from build123d import *

# Parameters (mm, degrees)
F1_DEPTH = 1


with BuildPart() as f1:
    # F0 (on Front) → F1 (new body)
    with BuildSketch(Plane.XZ):
        with BuildLine():
            Line((18.708066, 12.50033), (22.98097, 22.98097))
            Line((22.98097, 22.98097), (12.437212, 18.613602))
            Line((12.437212, 18.613602), (12.437212, 30.026085))
            Line((12.437212, 30.026085), (4.315137, 22.082337))
            Line((4.315137, 22.082337), (0, 32.5))
            Line((0, 32.5), (-4.371889, 22.071171))
            Line((-4.371889, 22.071171), (-12.359057, 30.058339))
            ThreePointArc((-12.359057, 30.058339), (-12.437212, 30.026085), (-12.515282, 29.993628))
            Line((-12.515282, 29.993628), (-12.515282, 18.730443))
            Line((-12.515282, 18.730443), (-22.921108, 23.040677))
            ThreePointArc((-22.921108, 23.040677), (-22.979929, 22.982012), (-23.0386, 22.923195))
            Line((-23.0386, 22.923195), (-18.623445, 12.626056))
            Line((-18.623445, 12.626056), (-29.947166, 12.626056))
            ThreePointArc((-29.947166, 12.626056), (-30.026085, 12.437212), (-30.103813, 12.247874))
            Line((-30.103813, 12.247874), (-22.096734, 4.240795))
            Line((-22.096734, 4.240795), (-32.499928, -0.068349))
            Line((-32.499928, -0.068349), (-22.067669, -4.389532))
            Line((-22.067669, -4.389532), (-30.052174, -12.374038))
            ThreePointArc((-30.052174, -12.374038), (-30.026085, -12.437212), (-29.999862, -12.50033))
            Line((-29.999862, -12.50033), (-18.708066, -12.50033))
            Line((-18.708066, -12.50033), (-23.02925, -22.93259))
            ThreePointArc((-23.02925, -22.93259), (-22.98097, -22.98097), (-22.93259, -23.02925))
            Line((-22.93259, -23.02925), (-12.50033, -18.708066))
            Line((-12.50033, -18.708066), (-12.50033, -29.999862))
            ThreePointArc((-12.50033, -29.999862), (-12.437212, -30.026085), (-12.374038, -30.052174))
            Line((-12.374038, -30.052174), (-4.389532, -22.067669))
            Line((-4.389532, -22.067669), (-0.068349, -32.499928))
            ThreePointArc((-0.068349, -32.499928), (0, -32.5), (0.068349, -32.499928))
            Line((0.068349, -32.499928), (4.389532, -22.067669))
            Line((4.389532, -22.067669), (12.437212, -30.026085))
            Line((12.437212, -30.026085), (12.437212, -18.613602))
            Line((12.437212, -18.613602), (22.98097, -22.98097))
            Line((22.98097, -22.98097), (18.613602, -12.437212))
            Line((18.613602, -12.437212), (30.026085, -12.437212))
            Line((30.026085, -12.437212), (22.033376, -4.558546))
            Line((22.033376, -4.558546), (32.499923, -0.070754))
            ThreePointArc((32.499923, -0.070754), (32.499981, -0.035377), (32.5, 0))
            ThreePointArc((32.5, 0), (32.499982, 0.034174), (32.499928, 0.068349))
            Line((32.499928, 0.068349), (22.067669, 4.389532))
            Line((22.067669, 4.389532), (30.052174, 12.374038))
            ThreePointArc((30.052174, 12.374038), (30.026085, 12.437212), (29.999862, 12.50033))
            Line((29.999862, 12.50033), (18.708066, 12.50033))
        make_face()
    extrude(amount=F1_DEPTH)


solid = f1.part
CAD build for the part. Positions are in the model's coordinates, mm. A direction names the side the tool comes from. Give positions to 0.01 mm unless a question says otherwise; leave off trailing zeros. Order: outer loops, then holes, each group sorted by start corner. A loop starts at its lowest first (then second) coordinate and runs counter-clockwise, first axis right, second up. Notation, with made-up numbers: (73.5, 54) -> (93.5, 54) arc R20 cw to (93.5, 62) -> close; hole circle Ø6 at (-23.75, 35). An arc over 180 degrees is marked (long way). Return JSON: item names as keys, results as strings.
Q1. Which spindle directions (+Z, -Z, +X, -X, +Y, -Y) get a long thin tool onto all of the face, cutting with end or side? Do faces 5 (the face through (-27.357, -0.493, -2.199)), 6 (the face through (2.199, -0.493, -27.357)), 7 (the face through (26.004, -0.493, 8.326)). Say none if no direction does.
Working result:
{"face 5": "-X, +Y, -Y", "face 6": "-Z, +Y, -Y", "face 7": "+X, +Y, -Y"}
Q2. Saw through at A-A (x = 25.5). Write the cut outline in (y, z).
Working result:
{"outline": "(-1, -12.44) -> (0, -12.44) -> (0, -7.98) -> (-1, -7.98) -> close; (-1, -3.07) -> (0, -3.07) -> (0, 2.97) -> (-1, 2.97) -> close; (-1, 7.82) -> (0, 7.82) -> (0, 12.5) -> (-1, 12.5) -> close"}
Q3. Drill centre lines: line 1 (X direction, y = -0.85, z = -28); line 2 (Z direction, x = -29, y = -0.9); line 3 (X direction, y = -0.45, z = 22.5). Where is each one in solid material? Low to high.
Working result:
{"line 1": "-12.5 to -10.32, -1.93 to 1.93, 10.39 to 12.44", "line 2": "-12.5 to -11.32, -1.52 to 1.38, 11.14 to 12.63", "line 3": "-22.86 to -21.62, -12.52 to -4.8, -4.19 to 4.14, 4.74 to 12.44, 21.82 to 22.78"}
Q4. Flat gauge pin, fed straight in: pin 1 (0.5 mm diameter, centred on y = -0.5, z = -26, fed in from -X). Where does the tip first touch, or does it go through?
Working result:
{"pin 1": "x = -12.5"}
Q5. Saw through at D-D (x = 10). Write the cut outline in (y, z), then the cut area to 3 significant figures.
Working result:
{"outline": "(-1, -27.62) -> (0, -27.62) -> (0, 27.64) -> (-1, 27.64) -> close", "area": "55.3 mm²"}
Q6. Saw through at B-B (x = -27). Write the cut outline in (y, z).
Working result:
{"outline": "(-1, -12.5) -> (0, -12.5) -> (0, -9.32) -> (-1, -9.32) -> close; (-1, -2.35) -> (0, -2.35) -> (0, 2.21) -> (-1, 2.21) -> close; (-1, 9.14) -> (0, 9.14) -> (0, 12.63) -> (-1, 12.63) -> close"}
Q7. Mould opens along Z. For faces 1 (the face through (-2.155, -0.493, 27.359)), 2 (the face through (0, 0, 0)), 3 (the face through (-2.26, -0.49, -27.21)), 4 (the face through (-26.156, -0.493, 8.3)) say: pulls with the +Z half, pulls with the -Z half, needs draft (parallel to the pull), parting line crosses it, or undercut.
Working result:
{"face 1": "pulls with the +Z half", "face 2": "needs draft", "face 3": "pulls with the -Z half", "face 4": "undercut"}
Q8. Saw through at C-C (z = -6). Write the cut outline in (x, y), then the cut area to 3 significant figures.
Working result:
{"outline": "(-23.68, -1) -> (23.5, -1) -> (23.5, 0) -> (-23.68, 0) -> close", "area": "47.2 mm²"}
